Geometry check sheet. Reference: the model listing, model coordinates, mm. A direction names the side the tool comes from. Coordinates: 2 decimals unless noted, no trailing zeros. Loops run counter-clockwise (first coordinate to the right, second up) from the corner with the lowest first, then second, coordinate; pieces in that order, holes last.
from build123d import *

# Parameters (mm, degrees)
F1_DEPTH       = 1174
F3_DEPTH       = 664
F4_W           = 40
F4_H           = 40
F5_DEPTH       = 4
F6_W           = 4
F6_H           = 4
F7_DEPTH       = 350
F8_R           = 2
F8_2_R         = 2
F8_3_R         = 2
F8_4_R         = 2
F10_DEPTH      = 21
F12_DEPTH      = 25
F12_DEPTH_BACK = 25
F15_D          = 5
F15_ON_F13_D   = 5


with BuildPart() as f1:
    # F0 (on Front) → F1 (new body)
    with BuildSketch(Plane.XZ):
        Polygon((38, -2), (38, -25), (40, -25), (40, 0), (0, 0), (0, -350), (27, -350), (27, -376), (29, -376), (29, -348), (2, -348), (2, -2), align=None)
    extrude(amount=F1_DEPTH)

    # F8
    f8_edges = [f1.edges().sort_by_distance(p)[0] for p in [
        (40, -587, 0),
        (29, -587, -348),
        (2, -587, -348),
        (0, -587, 0),
        (2, -587, -2),
        (38, -587, -2),
        (0, -587, -350),
        (27, -587, -350),
    ]]
    fillet(f8_edges, radius=F8_R)



with BuildPart() as f3:
    # F2 (on Right) → F3 (new body)
    with BuildSketch(Plane.YZ):
        Polygon((38, -2), (38, -25), (40, -25), (40, 0), (0, 0), (0, -350), (27, -350), (27, -376), (29, -376), (29, -348), (2, -348), (2, -2), align=None)
    extrude(amount=-F3_DEPTH)

    # F8#2
    f8_2_edges = [f3.edges().sort_by_distance(p)[0] for p in [
        (-332, 40, 0),
        (-332, 29, -348),
        (-332, 2, -348),
        (-332, 0, 0),
        (-332, 2, -2),
        (-332, 38, -2),
        (-332, 0, -350),
        (-332, 27, -350),
    ]]
    fillet(f8_2_edges, radius=F8_2_R)


with BuildPart() as f5:
    # F4 (on Top) → F5 (new body)
    with BuildSketch(Plane.XY):
        with Locations((20, 20)):
            Rectangle(F4_W, F4_H)
    extrude(amount=-F5_DEPTH)

    # F8#4
    f8_4_edges = [f5.edges().sort_by_distance(p)[0] for p in [
        (40, 20, 0),
        (20, 40, 0),
    ]]
    fillet(f8_4_edges, radius=F8_4_R)


with BuildPart() as f7:
    # F6 (on Top) → F7 (new body)
    with BuildSketch(Plane.XY):
        with Locations((2, 2)):
            Rectangle(F6_W, F6_H)
    extrude(amount=-F7_DEPTH)

    # F8#3
    f8_3_edges = [f7.edges().sort_by_distance(p)[0] for p in [
        (4, 4, -175),
    ]]
    fillet(f8_3_edges, radius=F8_3_R)


with BuildPart() as f10:
    # F9 (on face) → F10 (new body)
    with BuildSketch(Plane(origin=(0, 0, -4), x_dir=(1, 0, 0), z_dir=(0, 0, -1))):
        Polygon((40, -40), (40, 0), (36, 0), (36, -36), (0, -36), (0, -40), align=None)
    extrude(amount=F10_DEPTH)


with BuildPart() as f1_1:
    add(f1.part)

    add(f3.part)  # F12 merges F3

    add(f5.part)  # F12 merges F5

    add(f7.part)  # F12 merges F7

    add(f10.part)  # F12 merges F10
    # F11 (on face) → F12 (join, two sides)
    with BuildSketch(Plane.XZ.offset(1174)) as f12_sk:
        with BuildLine():
            Line((27, -346), (4, -346))
            Line((4, -346), (4, -4))
            Line((4, -4), (36, -4))
            Line((36, -4), (36, -25))
            Line((36, -25), (38, -25))
            Line((38, -25), (38, -4))
            ThreePointArc((38, -4), (37.4142135624, -2.5857864376), (36, -2))
            Line((36, -2), (4, -2))
            ThreePointArc((4, -2), (2.5857864376, -2.5857864376), (2, -4))
            Line((2, -4), (2, -346))
            ThreePointArc((2, -346), (2.5857864376, -347.4142135624), (4, -348))
            Line((4, -348), (27, -348))
            Line((27, -348), (27, -346))
        make_face()
    extrude(amount=F12_DEPTH)
    extrude(f12_sk.sketch, amount=-F12_DEPTH_BACK)

    # F15 (through all)
    with Locations(Plane(origin=(27, 0, 0), x_dir=(0, -1, 0), z_dir=(-1, 0, 0))):
        with Locations((100, -364), (587, -364), (1074, -364)):
            Hole(F15_D / 2)

    # F15 on F13 (through all)
    with Locations(Plane.XZ.offset(-27)):
        with Locations((-100, -364), (-332, -364), (-564, -364)):
            Hole(F15_ON_F13_D / 2)


solid = f1_1.part
(1) Sectioned sample at B-B on z = -95. Record the cut outline in (x, y), and give its area (3 significant figures).
Findings:
outline: (-664, 0) - (0, 0) - (0, -1174) - (2, -1174) - (2, -1199) - (4, -1199) - (4, -1149) - (2, -1149) - (2, 0) - (4, 0) - (4, 2) arc R2 ccw to (2, 4) - (0, 4) - (0, 2) - (-664, 2) - close
area: 3,790 mm2
(2) Scan lines: L1, parallel to Z at x = 28, y = -1074; L2, parallel to Z at x = 27.7, y = -587; L3, parallel to Y at x = -106.5, z = -184.5. Record each from-to range of solid material in increasing order.
Findings:
L1: z = -376 to -366.5, -361.5 to -348.27, -2 to 0
L2: z = -376 to -366.5, -361.5 to -348.13, -2 to 0
L3: y = 0 to 2
(3) Draft check along Z on faces 6 (the flat face through (20, -1186, -2)), 7 (the flat face through (14, -577, -350)), 8 (the flat face through (29, -579, -363)), 9 (the flat face through (-327, 2, -177)). Enter one of: +Z half, -Z half, draft (parallel to the pull), parting line (faces both ways), or undercut.
Findings:
face 6: +Z half
face 7: -Z half
face 8: draft
face 9: undercut
(4) Sectioned sample at A-A on x = -542. Record the cut outline in (y, z).
Findings:
outline: (0, -348) arc R2 ccw to (2, -350) - (25, -350) arc R2 cw to (27, -352) - (27, -376) - (29, -376) - (29, -350) arc R2 ccw to (27, -348) - (4, -348) arc R2 cw to (2, -346) - (2, -4) arc R2 cw to (4, -2) - (36, -2) arc R2 cw to (38, -4) - (38, -25) - (40, -25) - (40, -2) arc R2 ccw to (38, 0) - (2, 0) arc R2 ccw to (0, -2) - close
(5) Gauge pin test, flat ends, axial feed: pin 1 Ø2 at (x, z) = (-496, -335) entering from -Y; pin 2 Ø7.5 at (y, z) = (-1183, -215) entering from -X; pin 3 Ø12.5 at (x, y) = (26.5, -1192.5) entering from +Z; pin 4 Ø23 at (y, z) = (-1181.5, -13) entering from +X. Record the tip position at first contact, or that the pin passes through.
Findings:
pin 1: stops at y = 0
pin 2: stops at x = 2
pin 3: stops at z = -2
pin 4: stops at x = 40
(6) Access from +Z, -Z, +X, -X, +Y, -Y to the whole of each face (thin tool, end or side, straight path). Record for faces 1 (the flat face through (20, -1174, -4)), 2 (the flat face through (-327, 0, -173)), 3 (the flat face through (28, 0, -356)), 4 (the flat face through (-327, 29, -363)), 5 (the flat face through (27, -579, -364)).
Findings:
face 1: -Y
face 2: +Z, -Z, -X, -Y
face 3: -Z, +X, +Y
face 4: -Z, +X, -X, +Y
face 5: -Z, -X, +Y, -Y
